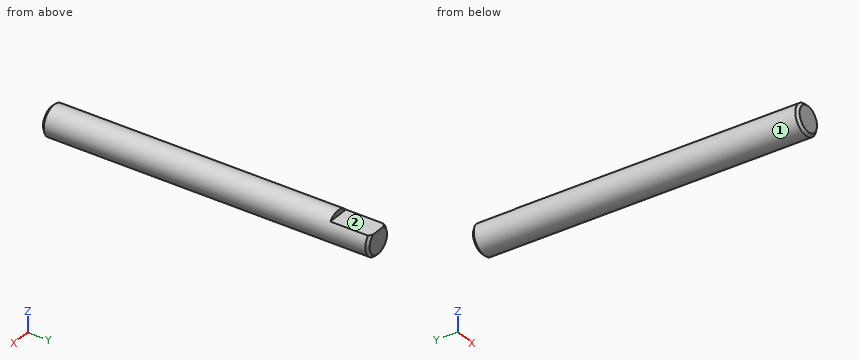
```python
from build123d import *

# Parameters (mm, degrees)
SKETCH1_R           = 3
BOSS_EXTRUDE1_DEPTH = 65
CUT_EXTRUDE1_DEPTH  = 8
CHAMFER1_SIZE       = 0.5


with BuildPart() as part:
    # Sketch1 → Boss-Extrude1 (new body)
    with BuildSketch(Plane(origin=(0, 0, 0), x_dir=(1, 0, 0), z_dir=(0, 1, 0))):
        Circle(SKETCH1_R)
    extrude(amount=BOSS_EXTRUDE1_DEPTH)

    # Sketch2 → Cut-Extrude1 (cut)
    with BuildSketch(Plane(origin=(0, 65, 0), x_dir=(1, 0, 0), z_dir=(0, 1, 0))):
        with BuildLine():
            Line((-2.236067977, -2), (2.236067977, -2))
            ThreePointArc((2.236067977, -2), (0, -3), (-2.236067977, -2))
        make_face()
    extrude(amount=-CUT_EXTRUDE1_DEPTH, mode=Mode.SUBTRACT)

    # Chamfer1
    chamfer1_edges = [part.edges().sort_by_distance(p)[0] for p in [
        (-3, 0, 0),
        (-1.070466269, 65, -2.802517077),
    ]]
    chamfer(chamfer1_edges, length=CHAMFER1_SIZE)


solid = part.part
```
The listing builds one solid part. Answer for the finished solid, in the listing's coordinates (mm). Face numbers are marked on the shaded views. A direction names the side the tool comes from. Round coordinates to 2 decimals unless told otherwise and drop trailing zeros. Order: outer loops, then holes, each group sorted by start corner. A loop starts at its lowest first (then second) coordinate and runs counter-clockwise, first axis right, second up. Notation, with made-up numbers: (29.5, 21.5) -> (66.5, 21.5) arc R8 ccw to (66.5, 25.5) -> close; hole circle Ø6 at (60, 72). An arc over 180 degrees is marked (long way). Answer as CSV lines item,"result". Start each with the question number.
(1) The part is cut by section B-B (y = 12). Determine the outline of the cut face in (x, z).
(2) The part is cut by section A-A (x = 0). Determine the outline of the cut face in (y, z).
(3) A tool of negligible diameter and unlimited length cuts with its end or side. For the marked faces 1 and 2, from which of +Z, -Z, +X, -X, +Y, -Y can it reach the whole face along a straight path? Write none if from no direction.
(4) Flat-ended cylindrical pins translate along their axes: pin 1 Ø1.5 at (y, z) = (35.5, -2) entering from -X; pin 2 Ø0.8 at (x, z) = (-0.5, 2.5) entering from +Y; pin 3 Ø1.3 at (x, y) = (-0.5, 62.5) entering from +Z. Find the tip coordinate at first contact, or state that the pin passes through.
(5) Find the intervals of material crossed by probe 1 along Z at (x, y) = (-0.2, 61); probe 2 along X at (y, z) = (57.5, 0.15); probe 3 along Y at (x, z) = (-1.95, 1.6), in increasing order. Write a range as from..to.
Evaluation:
1,outline,"circle Ø6 at (0, 0)"
2,outline,"(0, -2.5) -> (0.5, -3) -> (64.5, -3) -> (65, -2.5) -> (65, 2) -> (57, 2) -> (57, 3) -> (0.5, 3) -> (0, 2.5) -> close"
3,face 1,"+Y, -Y"
3,face 2,"+Z, +X, -X, +Y"
4,pin 1,"x = -2.73"
4,pin 2,"y = 57"
4,pin 3,"z = 2"
5,probe 1,"-2.99..2"
5,probe 2,"-3..3"
5,probe 3,"0.02..64.98"
